Geometry check sheet. Reference: the model listing, model coordinates, mm. A direction names the side the tool comes from. Round coordinates to 2 decimals unless told otherwise and drop trailing zeros. Loops run counter-clockwise (first coordinate to the right, second up) from the corner with the lowest first, then second, coordinate; pieces in that order, holes last. Notation, with made-up numbers: M 50.5,-4.75 L 67.5,-4.75 A4 cw 67.5,0.25 Z; hole C 32.5,44 d4. An arc over 180 degrees is marked long. Use one line per item in the form item = value. Start each with the question number.
1. Cross-section at A-A (z = -9.75). Record the boundary of the cut face in (x, y), then the cut area to 3 significant figures.
2. Set-up check for faces 1 (the flat face through (0, 0, 8)), 2 (the flat face through (0, 11, -2)): record each of +Z, -Z, +X, -X, +Y, -Y from which the full face is reachable in a straight line by a thin tool's end or side.
3. Cross-section at C-C (x = 6). Record the boundary of the cut face in (y, z) (3 decimals), then the cut area to 3 significant figures.
4. Material ranges on line 1 (X direction, y = 8.5, z = -9.75); line 2 (Z direction, x = -17.5, y = 2.75) (3 decimals); line 3 (X direction, y = 8.5, z = 8.25), recorded low to high.
5. Cross-section at D-D (y = 12.75). Record the boundary of the cut face in (x, z), then the cut area to 3 significant figures.
6. Cross-section at B-B (y = 9.25). State how many separate pieces and enclosed holes the cut face has, then the cut area to 3 significant figures.
7. Go/stop test with a flat-tipped pin: pin 1 (1.5 mm diameter, centred on y = 12, z = 11, fed in from +X). Record where the tip stops, or that it passes through.
```python
from build123d import *

# Parameters (mm, degrees)
CROQUIS1_W              = 52
CROQUIS1_H              = 28
CROQUIS1_R              = 1.55
SALIENTE_EXTRUIR1_DEPTH = 14
CROQUIS2_W              = 62.635554568
CROQUIS2_H              = 10.05
CORTAR_EXTRUIR1_DEPTH   = 11
REDONDEO2_START         = -14
REDONDEO2_DEPTH         = 28
REDONDEO2_START_2       = -27
REDONDEO2_2_DEPTH       = 54
REDONDEO3_R             = 3


with BuildPart() as part:
    # Croquis1 → Saliente-Extruir1 (new body)
    with BuildSketch(Plane(origin=(0, 0, 0), x_dir=(1, 0, 0), z_dir=(0, 1, 0))):
        Rectangle(CROQUIS1_W, CROQUIS1_H)
        with Locations(Location((-21.372490304, -8.249987757, 0), (0, 0, 270))):
            Circle(CROQUIS1_R, mode=Mode.SUBTRACT)
        with Locations(Location((22.010248646, -8.249987757, 0), (0, 0, 270))):
            Circle(CROQUIS1_R, mode=Mode.SUBTRACT)
        with Locations(Location((-21.351495904, 9.75, 0), (0, 0, 270))):
            Circle(CROQUIS1_R, mode=Mode.SUBTRACT)
        with Locations(Location((21.989254247, 9.75, 0), (0, 0, 270))):
            Circle(CROQUIS1_R, mode=Mode.SUBTRACT)
    extrude(amount=SALIENTE_EXTRUIR1_DEPTH)

    # Croquis2 → Cortar-Extruir1 (cut)
    with BuildSketch(Plane.XZ):
        with Locations((0, -2.1)):
            Rectangle(CROQUIS2_W, CROQUIS2_H)
    extrude(amount=-CORTAR_EXTRUIR1_DEPTH, mode=Mode.SUBTRACT)

    # Redondeo2: read off the stored shape, not the designer's step
    # Redondeo2 outline → Redondeo2 (cut)
    with BuildSketch(Plane.XY.offset(REDONDEO2_START)):
        with BuildLine():
            ThreePointArc((-26, 11), (-25.121320344, 13.121320344), (-23, 14))
            Line((-23, 14), (-26, 14))
            Line((-26, 14), (-26, 11))
        make_face()
        with BuildLine():
            ThreePointArc((23, 14), (25.121320344, 13.121320344), (26, 11))
            Line((26, 11), (26, 14))
            Line((26, 14), (23, 14))
        make_face()
    extrude(amount=REDONDEO2_DEPTH, mode=Mode.SUBTRACT)

    # Redondeo2 2 outline → Redondeo2 2 (cut)
    with BuildSketch(Plane.YZ.offset(REDONDEO2_START_2)):
        with BuildLine():
            ThreePointArc((11, 14), (13.121320344, 13.121320344), (14, 11))
            Line((14, 11), (14, 14))
            Line((14, 14), (11, 14))
        make_face()
        with BuildLine():
            ThreePointArc((14, -11), (13.121320344, -13.121320344), (11, -14))
            Line((11, -14), (14, -14))
            Line((14, -14), (14, -11))
        make_face()
    extrude(amount=REDONDEO2_2_DEPTH, mode=Mode.SUBTRACT)

    # Redondeo3
    # the kernel refuses this fillet: 3 mm, written as the material it takes off along each edge
    with BuildSketch(Plane(origin=(23, 11, -11), x_dir=(1, 0, 0), z_dir=(0, 0, -1))) as redondeo3_piece_1_section:
        Polygon((0, 0), (REDONDEO3_R, 0), (REDONDEO3_R, -REDONDEO3_R), (0, -REDONDEO3_R), align=None)
    redondeo3_piece_1 = extrude(amount=REDONDEO3_R, mode=Mode.PRIVATE)
    redondeo3_piece_1 = redondeo3_piece_1 - Plane(origin=(23, 11, -11), x_dir=(-0.7071067811865475, -0.7071067811865475, 0), z_dir=(0, 0, -1)) * Sphere(REDONDEO3_R, mode=Mode.PRIVATE)
    add(redondeo3_piece_1, mode=Mode.SUBTRACT)
    with BuildSketch(Plane(origin=(23, 11, 11), x_dir=(0, 0, 1), z_dir=(1, 0, 0))) as redondeo3_piece_2_section:
        Polygon((0, 0), (REDONDEO3_R, 0), (REDONDEO3_R, -REDONDEO3_R), (0, -REDONDEO3_R), align=None)
    redondeo3_piece_2 = extrude(amount=REDONDEO3_R, mode=Mode.PRIVATE)
    redondeo3_piece_2 = redondeo3_piece_2 - Plane(origin=(23, 11, 11), x_dir=(0, -0.7071067811865475, -0.7071067811865475), z_dir=(1, 0, 0)) * Sphere(REDONDEO3_R, mode=Mode.PRIVATE)
    add(redondeo3_piece_2, mode=Mode.SUBTRACT)
    with BuildSketch(Plane(origin=(-23, 11, -11), x_dir=(-1, 0, 0), z_dir=(0, 0, -1))) as redondeo3_piece_3_section:
        Polygon((0, 0), (REDONDEO3_R, 0), (REDONDEO3_R, REDONDEO3_R), (0, REDONDEO3_R), align=None)
    redondeo3_piece_3 = extrude(amount=REDONDEO3_R, mode=Mode.PRIVATE)
    redondeo3_piece_3 = redondeo3_piece_3 - Plane(origin=(-23, 11, -11), x_dir=(0.7071067811865475, -0.7071067811865475, 0), z_dir=(0, 0, -1)) * Sphere(REDONDEO3_R, mode=Mode.PRIVATE)
    add(redondeo3_piece_3, mode=Mode.SUBTRACT)
    with BuildSketch(Plane(origin=(-23, 11, 11), x_dir=(0, 0, 1), z_dir=(-1, 0, 0))) as redondeo3_piece_4_section:
        Polygon((0, 0), (REDONDEO3_R, 0), (REDONDEO3_R, REDONDEO3_R), (0, REDONDEO3_R), align=None)
    redondeo3_piece_4 = extrude(amount=REDONDEO3_R, mode=Mode.PRIVATE)
    redondeo3_piece_4 = redondeo3_piece_4 - Plane(origin=(-23, 11, 11), x_dir=(0, -0.7071067811865475, -0.7071067811865475), z_dir=(-1, 0, 0)) * Sphere(REDONDEO3_R, mode=Mode.PRIVATE)
    add(redondeo3_piece_4, mode=Mode.SUBTRACT)
    with BuildSketch(Plane(origin=(-26, -7.5, 14), x_dir=(0, 0, -1), z_dir=(0, 1, 0)), Plane(origin=(-26, -7.5, -14), x_dir=(1, 0, 0), z_dir=(0, 1, 0))) as redondeo3_piece_5:
        with BuildLine():
            CenterArc((REDONDEO3_R, -REDONDEO3_R), REDONDEO3_R, 90, 90)
            Line((0, -REDONDEO3_R), (0, 0))
            Line((0, 0), (REDONDEO3_R, 0))
        make_face()
    extrude(amount=18.5, mode=Mode.SUBTRACT)
    with BuildSketch(Plane(origin=(26, -7.5, -14), x_dir=(-1, 0, 0), z_dir=(0, 1, 0)), Plane(origin=(26, -7.5, 14), x_dir=(0, 0, -1), z_dir=(0, 1, 0))) as redondeo3_piece_6:
        with BuildLine():
            CenterArc((REDONDEO3_R, REDONDEO3_R), REDONDEO3_R, 180, 90)
            Line((0, REDONDEO3_R), (0, 0))
            Line((0, 0), (REDONDEO3_R, 0))
        make_face()
    extrude(amount=18.5, mode=Mode.SUBTRACT)


solid = part.part
```
Reported:
q1.outline = M -26,0 L -22.9,0 L -22.9,14 L -23,14 A3 ccw -26,11 Z; M -19.8,0 L 20.44,0 L 20.44,14 L -19.8,14 Z; M 23.54,0 L 26,0 L 26,11 A3 ccw 23.54,13.95 Z
q1.area = 637 mm²
q2.face_1 = +Z, -Z, +X, -X, -Y
q2.face_2 = +X, -X, -Y
q3.outline = M 0,-14 L 11,-14 A3 ccw 14,-11 L 14,11 A3 ccw 11,14 L 0,14 L 0,2.925 L 11,2.925 L 11,-7.125 L 0,-7.125 Z
q3.area = 278 mm²
q4.line_1 = -26 to -22.9, -19.8 to 20.44, 23.54 to 26
q4.line_2 = -14 to -7.125, 2.925 to 14
q4.line_3 = -26 to -22.92, -19.82 to 20.46, 23.56 to 26
q5.outline = M -25.44,-11 A2.44 ccw -23,-13.44 L 23,-13.44 A2.44 ccw 25.44,-11 L 25.44,11 A2.44 ccw 23,13.44 L -23,13.44 A2.44 ccw -25.44,11 Z; hole C -21.37,8.25 d3.1; hole C -21.35,-9.75 d3.1; hole C 21.99,-9.75 d3.1; hole C 22.01,8.25 d3.1
q5.area = 1,330 mm²
q6.separate_pieces = 2
q6.enclosed_holes = 4
q6.area = 895 mm²
q7.pin_1 = 25.99
